from build123d import *

# Parameters (mm, degrees)
SKETCH1_W          = 76.2
SKETCH1_H          = 6.35
BASE_EXTRUDE_DEPTH = 19.05
CUT_EXTRUDE1_DEPTH = 7.35
SKETCH3_R          = 2.38125
CUT_EXTRUDE2_DEPTH = 7.35


with BuildPart() as part:
    # Sketch1 → Base-Extrude (new body)
    with BuildSketch(Plane.XY):
        with Locations((38.1, 3.175)):
            Rectangle(SKETCH1_W, SKETCH1_H)
    extrude(amount=BASE_EXTRUDE_DEPTH)

    # Sketch2 → Cut-Extrude1 (cut, through all)
    with BuildSketch(Plane(origin=(0, 6.35, 0), x_dir=(-1, 0, 0), z_dir=(0, 1, 0))):
        with BuildLine():
            Line((-71.5645, 5.473421326), (-71.5645, 13.576578674))
            ThreePointArc((-71.5645, 13.576578674), (-60.325, 9.525), (-71.5645, 5.473421326))
        make_face()
    extrude(amount=-CUT_EXTRUDE1_DEPTH, mode=Mode.SUBTRACT)

    # Sketch3 → Cut-Extrude2 (cut, through all)
    with BuildSketch(Plane(origin=(0, 6.35, 0), x_dir=(-1, 0, 0), z_dir=(0, 1, 0))):
        with Locations((-9.525, 9.525)):
            Circle(SKETCH3_R)
    extrude(amount=-CUT_EXTRUDE2_DEPTH, mode=Mode.SUBTRACT)


solid = part.part
Part model, mm, in its own coordinate system. Coordinates: 2 decimals unless noted, no trailing zeros. Loops run counter-clockwise (first coordinate to the right, second up) from the corner with the lowest first, then second, coordinate; pieces in that order, holes last. Notation, with made-up numbers: M 42,-3.75 L 91,-3.75 A29 ccw 91,27.25 Z; hole C 38,76.5 d4. An arc over 180 degrees is marked long. Use a Markdown table: item, result. Add a question column.
Q1. Cut at A-A (y = 1.5). Give the number of separate pieces and of enclosed holes in the cut face, and give its area (3 significant figures).
Q2. Cut at B-B (x = 65). Write the cut outline in (y, z).
Q3. Pin check, flat tip, straight feed: P1, Ø1, axis at x = 29, z = 8.5, coming from the -Y side. Stop position of the tip, or through.
Q4. Mould opens along Z. For faces 1 (the flat face through (38, 0, 9)), 2 (the flat face through (38, 3, 19.05)), 3 (the flat face through (71.564, 3, 9)), 4 (the flat face through (38, 3, 0)) say: +Z half, -Z half, draft (parallel to the pull), parting line (faces both ways), or undercut.
Q5. Probe L1, parallel to X at y = 3, z = 9.25; L2, parallel to X at y = 5.25, z = 7.75; L3, parallel to Z at x = 9.5, y = 1. List the from-to ranges inside material, lowest first.
Worked out:
| question | item | result |
|---|---|---|
| 1 | separate pieces | 1 |
| 1 | enclosed holes | 2 |
| 1 | area | 1,320 mm2 |
| 2 | outline | M 0,0 L 6.35,0 L 6.35,3.4 L 0,3.4 Z; M 0,15.65 L 6.35,15.65 L 6.35,19.05 L 0,19.05 Z |
| 3 | P1 | stops at y = 0 |
| 4 | face 1 | draft |
| 4 | face 2 | +Z half |
| 4 | face 3 | undercut |
| 4 | face 4 | -Z half |
| 5 | L1 | x = 0 to 7.16, 11.89 to 60.33, 71.56 to 76.2 |
| 5 | L2 | x = 0 to 7.94, 11.11 to 60.58, 71.56 to 76.2 |
| 5 | L3 | z = 0 to 7.14, 11.91 to 19.05 |
